from build123d import *

# Parameters (mm, degrees)
SKETCH1_W               = 45
SKETCH1_H               = 85
BOSS_EXTRUDE1_DEPTH     = 100
SHELL1_T                = -5
SKETCH2_W               = 3
SKETCH2_H               = 10
BOSS_EXTRUDE2_DEPTH     = 15
SKETCH4_W               = 20
SKETCH4_H               = 2.5
BOSS_EXTRUDE3_DEPTH     = 1
SKETCH5_W               = 13.798148254
SKETCH5_H               = 2.5
BOSS_EXTRUDE4_DEPTH     = 1
SKETCH6_W               = 10
SKETCH6_H               = 2.5
BOSS_EXTRUDE5_DEPTH     = 1
SKETCH9_W               = 10.477527882
SKETCH9_H               = 6.322646136
CUT_EXTRUDE1_DEPTH      = 11
CUT_EXTRUDE2_DEPTH      = 107.477697195
CUT_EXTRUDE2_DEPTH_BACK = 107.477697195
SKETCH10_W              = 54.233150032
SKETCH10_H              = 93.874108495
SKETCH10_W_2            = 30
SKETCH10_H_2            = 50


with BuildPart() as part:
    # Sketch1 → Boss-Extrude1 (new body)
    with BuildSketch(Plane(origin=(0, 0, 0), x_dir=(1, 0, 0), z_dir=(0, 1, 0))):
        Rectangle(SKETCH1_W, SKETCH1_H)
    extrude(amount=BOSS_EXTRUDE1_DEPTH)

    # Shell1
    shell1_openings = [part.faces().sort_by_distance(p)[0] for p in [
        (0, 100, 0),
    ]]
    offset(amount=SHELL1_T, openings=shell1_openings, kind=Kind.INTERSECTION)

    # Sketch2 → Boss-Extrude2 (add)
    with BuildSketch(Plane(origin=(0, 5, 0), x_dir=(1, 0, 0), z_dir=(0, 1, 0))):
        with BuildLine():
            Line((-13.25, -30), (-13.25, -25))
            Line((-13.25, -25), (-16.25, -25))
            Line((-16.25, -25), (-16.25, -33))
            Line((-16.25, -33), (1.75, -33))
            Line((1.75, -33), (1.75, -16.155494421))
            ThreePointArc((1.75, -16.155494421), (0.251072202, -16.248060277), (-1.25, -16.201851746))
            Line((-1.25, -16.201851746), (-1.25, -30))
            Line((-1.25, -30), (-13.25, -30))
        make_face()
        with Locations((-14.75, -20)):
            Rectangle(SKETCH2_W, SKETCH2_H)
        with BuildLine():
            Line((-16.25, -15), (-13.25, -15))
            Line((-13.25, -15), (-13.25, -9.407443861))
            ThreePointArc((-13.25, -9.407443861), (-15.481844205, -4.937104415), (-16.25, 0))
            Line((-16.25, 0), (-16.25, -15))
        make_face()
        with BuildLine():
            Line((-4.205809483, 15.696294677), (-3.429352348, 12.798517198))
            ThreePointArc((-3.429352348, 12.798517198), (0, 13.25), (3.429352348, 12.798517198))
            Line((3.429352348, 12.798517198), (4.205809483, 15.696294677))
            ThreePointArc((4.205809483, 15.696294677), (0, 16.25), (-4.205809483, 15.696294677))
        make_face()
        with BuildLine():
            ThreePointArc((-16.25, 0), (-15.481844205, -4.937104415), (-13.25, -9.407443861))
            Line((-13.25, -9.407443861), (-13.25, 0))
            Line((-13.25, 0), (-16.25, 0))
        make_face()
    extrude(amount=BOSS_EXTRUDE2_DEPTH)

    # Sketch4 → Boss-Extrude3 (add)
    with BuildSketch(Plane(origin=(-13.25, 0, 0), x_dir=(0, 0, -1), z_dir=(1, 0, 0))):
        with Locations((-20, 18.75)):
            Rectangle(SKETCH4_W, SKETCH4_H)
    extrude(amount=BOSS_EXTRUDE3_DEPTH)

    # Sketch5 → Boss-Extrude4 (add)
    with BuildSketch(Plane.ZY.offset(1.25)):
        with Locations((23.100925873, 18.75)):
            Rectangle(SKETCH5_W, SKETCH5_H)
    extrude(amount=BOSS_EXTRUDE4_DEPTH)

    # Sketch6 → Boss-Extrude5 (add)
    with BuildSketch(Plane(origin=(0, 0, 30), x_dir=(-1, 0, 0), z_dir=(0, 0, -1))):
        with Locations((7.25, 18.75)):
            Rectangle(SKETCH6_W, SKETCH6_H)
    extrude(amount=BOSS_EXTRUDE5_DEPTH)

    # Sketch9 → Cut-Extrude1 (cut)
    with BuildSketch(Plane(origin=(0, 20, 0), x_dir=(1, 0, 0), z_dir=(0, 1, 0))):
        with Locations((0.163497959, 14.216347227)):
            Rectangle(SKETCH9_W, SKETCH9_H)
    extrude(amount=-CUT_EXTRUDE1_DEPTH, mode=Mode.SUBTRACT)

    # Sketch10 → Cut-Extrude2 (cut, two sides: drawn at the far end of the back side and taken through both)
    with BuildSketch(Plane(origin=(0, 5, 0), x_dir=(1, 0, 0), z_dir=(0, 1, 0)).offset(-CUT_EXTRUDE2_DEPTH_BACK)):
        with Locations((1.369563357, 1.0979216)):
            Rectangle(SKETCH10_W, SKETCH10_H)
        with Locations((-1.25, -8)):
            Rectangle(SKETCH10_W_2, SKETCH10_H_2, mode=Mode.SUBTRACT)
    extrude(amount=CUT_EXTRUDE2_DEPTH + CUT_EXTRUDE2_DEPTH_BACK, mode=Mode.SUBTRACT)


solid = part.part
Can you work these out from the model? Positions are in its coordinate system, mm. A direction names the side the tool comes from. Give positions to 0.01 mm unless a question says otherwise; leave off trailing zeros. Order: outer loops, then holes, each group sorted by start corner. A loop starts at its lowest first (then second) coordinate and runs counter-clockwise, first axis right, second up. Notation, with made-up numbers: M -17,51 L 41,51 A12 cw 41,60 Z; hole C -5,-39 d10. An arc over 180 degrees is marked long. One line per item, written item: value.
Item 1: If we section it at B-B on x = -5: Write out the boundary of the cut face in (y, z), and give its area (4 significant figures).
Verdict:
outline: M 0,-17 L 5,-17 L 5,30 L 17.5,30 L 17.5,29 L 20,29 L 20,33 L 0,33 Z
area: 297.5 mm2
Item 2: If we section it at D-D on y = 15.25: Write out the boundary of the cut face in (x, z), and give its area (3 significant figures).
Verdict:
outline: M -16.25,0 L -13.25,0 L -13.25,30 L -1.25,30 L -1.25,16.2 A16.25 cw 1.75,16.16 L 1.75,33 L -16.25,33 Z
area: 185 mm2
Item 3: If we mould it in two halves opening along Y, with no side actions, what happens to faces 5 (the face through (-13.25, 12, 15)), 6 (the face through (-1, 0, 8)), 7 (the face through (-16.25, 10, 14))? For each: pulls with the +Y half, pulls with the -Y half, needs draft (parallel to the pull), parting line crosses it, or undercut.
Verdict:
face 5: undercut
face 6: pulls with the -Y half
face 7: needs draft
Item 4: For faces 1 (the face through (-0.05, 6.97, -13.25)), 2 (the face through (1.75, 12, 25)), 3 (the face through (-7, 19, 29)), 4 (the face through (-1.25, 11, 23)), which set-ups out of +Z, -Z, +X, -X, +Y, -Y let a thin tool reach every point of the face, with its end or its side?
Verdict:
face 1: +Y
face 2: +Z, +X, +Y
face 3: -Z, +Y
face 4: none
Item 5: Please list where these lines run through material, in increasing order: line 1 (X direction, y = 6.25, z = 24); line 2 (X direction, y = 16, z = 1); line 3 (X direction, y = 18.75, z = 18.5).
Verdict:
line 1: -16.25 to -13.25, -1.25 to 1.75
line 2: -16.25 to -13.25
line 3: -16.25 to -12.25, -2.25 to 1.75
Item 6: If we section it at A-A on y = 8.5: Write out the boundary of the cut face in (x, z).
Verdict:
outline: M -16.25,0 L -13.25,0 L -13.25,30 L -1.25,30 L -1.25,16.2 A16.25 cw 1.75,16.16 L 1.75,33 L -16.25,33 Z; M -4.21,-15.7 A16.25 ccw 4.21,-15.7 L 3.43,-12.8 A13.25 cw -3.43,-12.8 Z
Item 7: For pin 1 (4.5 mm diameter, centred on y = 12.5, z = 20, fed in from +X); pin 2 (1.5 mm diameter, centred on y = 10, z = -0.5, fed in from +X); pin 3 (13 mm diameter, centred on x = -7, z = 21, fed in from -Y); pin 4 (0.9 mm diameter, centred on x = -14.5, y = 10, fed in from -Z), each with a flat end and sliding along its axis, tell me the tip position at first contact or that it passes through.
Verdict:
pin 1: x = 1.75
pin 2: x = -13.25
pin 3: y = 0
pin 4: z = 0
Item 8: If we section it at C-C on z = 23.5: Write out the boundary of the cut face in (x, y), and give its area (3 significant figures).
Verdict:
outline: M -16.25,0 L 13.75,0 L 13.75,5 L 1.75,5 L 1.75,20 L -2.25,20 L -2.25,17.5 L -1.25,17.5 L -1.25,5 L -13.25,5 L -13.25,17.5 L -12.25,17.5 L -12.25,20 L -16.25,20 Z
area: 245 mm2
